Work out the finished part from the listing and answer in its coordinate system (mm). Coordinates: 2 decimals unless noted, no trailing zeros. Order: outer loops, then holes, each group sorted by start corner. A loop starts at its lowest first (then second) coordinate and runs counter-clockwise, first axis right, second up. Notation, with made-up numbers: (65.5, -9) -> (115.5, -9) arc R12 ccw to (115.5, -2) -> close; hole circle Ø11 at (64.25, 3.5). An arc over 180 degrees is marked (long way). Write item = value, one per line. Start each with the question number.
Q1. Flat-ended cylindrical pins translate along their axes: pin 1 (5 mm diameter, centred on y = 52, z = 9, fed in from +X); pin 2 (6 mm diameter, centred on x = 43.5, y = -23, fed in from -Z); pin 3 (3 mm diameter, centred on x = 52.5, z = 9.5, fed in from +Y); pin 4 (7.5 mm diameter, centred on y = 58.5, z = 7.5, fed in from +X). Find the tip coordinate at first contact, or state that the pin passes through.
Q2. Straight lines are drawn through the part: L1, parallel to X at y = -16, z = 5; L2, parallel to Y at x = 8, z = 11; L3, parallel to Y at x = 56, z = 4. For each, find the intervals that lie inside material, in ascending order. Write a range as from..to.
Q3. The part is cut by section A-A, the plane z = 2.75. Count the separate pieces of the cut face and the enclosed holes in it, plus the area to 3 significant figures.
Q4. For a pull along X with two mould halves and no side action, classify faces 1 (the flat face through (40.004, -48.798, 6.261)), 2 (the flat face through (16, 1, 12.7)), 3 (the flat face through (-12.11, -6.2, 6.26)) as +X half, -X half, draft (parallel to the pull), parting line (faces both ways), or undercut.
Q5. The part is cut by section C-C, the plane y = 33.5. Determine the outline of the cut face in (x, z).
Q6. The part is cut by section B-B, the plane x = -16.5. Determine the outline of the cut face in (y, z), plus the area to 3 significant figures.
```python
from build123d import *

# Parameters (mm, degrees)
F0_R     = 76.4587467439
F1_DEPTH = 12.7


with BuildPart() as f1:
    # F0 (on Top) → F1 (new body)
    with BuildSketch(Plane.XY):
        Circle(F0_R)
        with BuildLine():
            ThreePointArc((0, 67.8734653551), (47.9937876152, 47.9937876152), (67.8734653551, 0))
            ThreePointArc((67.8734653551, 0), (-31.0463451655, -60.3567042769), (-39.4713337388, 55.2161309057))
            Line((-39.4713337388, 55.2161309057), (-39.3394193415, 55.5124154929))
            Line((-39.3394193415, 55.5124154929), (-39.0032717993, 55.5477460232))
            ThreePointArc((-39.0032717993, 55.5477460232), (-20.4522527371, 64.7187195276), (0, 67.8734653551))
        make_face(mode=Mode.SUBTRACT)
        with BuildLine():
            ThreePointArc((-39.4713337388, 55.2161309057), (-31.0463451655, -60.3567042769), (67.8734653551, 0))
            ThreePointArc((67.8734653551, 0), (47.9937876152, 47.9937876152), (0, 67.8734653551))
            ThreePointArc((0, 67.8734653551), (-20.4522527371, 64.7187195276), (-39.0032717993, 55.5477460232))
            Line((-39.0032717993, 55.5477460232), (-29.885018528, 56.5061130603))
            Line((-29.885018528, 56.5061130603), (-24.2972507842, 48.8152105619))
            Line((-24.2972507842, 48.8152105619), (-28.1638838539, 40.1306104961))
            Line((-28.1638838539, 40.1306104961), (-37.6182846674, 39.1369129287))
            Line((-37.6182846674, 39.1369129287), (-43.2060524113, 46.8278154271))
            Line((-43.2060524113, 46.8278154271), (-39.4713337388, 55.2161309057))
        make_face()
        Polygon((-30.9335204728, -53.4327342282), (-40.3879212864, -52.4390366608), (-44.2545543561, -43.754436595), (-38.6667866123, -36.0635340966), (-29.2123857987, -37.057231664), (-25.345752729, -45.7418317298), align=None, mode=Mode.SUBTRACT)
        Polygon((6.9368320268, -60.8086286285), (-1.2960196783, -65.5618677767), (-9.5288713835, -60.8086286285), (-9.5288713835, -51.3021503321), (-1.2960196783, -46.548911184), (6.9368320268, -51.3021503321), align=None, mode=Mode.SUBTRACT)
        Polygon((-57.235837277, -25.2058756113), (-64.3005274315, -18.8448000245), (-62.3240194552, -9.5460610875), (-53.2828213244, -6.6083977373), (-46.21813117, -12.969473324), (-48.1946391463, -22.268212261), align=None, mode=Mode.SUBTRACT)
        Polygon((41.9100327329, -44.5162178486), (38.0433996632, -53.2008179144), (28.5889988496, -54.1945154818), (23.0012311058, -46.5036129834), (26.8678641755, -37.8190129176), (36.3222649891, -36.8253153502), align=None, mode=Mode.SUBTRACT)
        Polygon((60.6275076712, -10.7786490478), (62.6040156475, -20.0773879848), (55.539325493, -26.4384635716), (46.4981273623, -23.5008002214), (44.521619386, -14.2020612844), (51.5863095404, -7.8409856976), align=None, mode=Mode.SUBTRACT)
        Polygon((-61.9235273495, 13.0902466263), (-63.9000353258, 22.3889855633), (-56.8353451714, 28.7500611501), (-47.7941470406, 25.8123977998), (-45.8176390643, 16.5136588628), (-52.8823292188, 10.1525832761), align=None, mode=Mode.SUBTRACT)
        Polygon((4.2561218167, 13.0989960474), (8.0956247758, 11.1426715763), (11.1426715763, 8.0956247758), (13.0989960474, 4.2561218167), (13.7730995193, 0), (13.0989960474, -4.2561218167), (11.1426715763, -8.0956247758), (8.0956247758, -11.1426715763), (4.2561218167, -13.0989960474), (0, -13.7730995193), (-4.2561218167, -13.0989960474), (-8.0956247758, -11.1426715763), (-11.1426715763, -8.0956247758), (-13.0989960474, -4.2561218167), (-13.7730995193, 0), (-13.0989960474, 4.2561218167), (-11.1426715763, 8.0956247758), (-8.0956247758, 11.1426715763), (-4.2561218167, 13.0989960474), (0, 13.7730995193), align=None, mode=Mode.SUBTRACT)
        Polygon((55.9398175987, 27.5174731897), (63.0045077531, 21.156397603), (61.0279997768, 11.857658666), (51.9868016461, 8.9199953157), (44.9221114916, 15.2810709025), (46.8986194679, 24.5798098395), align=None, mode=Mode.SUBTRACT)
        Polygon((29.6375007945, 55.7443318067), (39.091901608, 54.7506342393), (42.9585346778, 46.0660341735), (37.3707669339, 38.3751316751), (27.9163661204, 39.3688292425), (24.0497330506, 48.0534293083), align=None, mode=Mode.SUBTRACT)
        Polygon((-8.2328517052, 63.1202262069), (0, 67.8734653551), (8.2328517052, 63.1202262069), (8.2328517052, 53.6137479106), (0, 48.8605087624), (-8.2328517052, 53.6137479106), align=None, mode=Mode.SUBTRACT)
    extrude(amount=F1_DEPTH)


solid = f1.part
```
Model answer:
q1.pin_1 = 58.27
q1.pin_2 = 0
q1.pin_3 = 56.96
q1.pin_4 = 53.37
q2.L1 = -74.77..-63.7, -46.86..44.9, 61.74..74.77
q2.L2 = -76.04..-11.19, 11.19..53.48, 63.25..76.04
q2.L3 = -52.06..-26.02, -9.28..10.22, 27.46..52.06
q3.separate_pieces = 1
q3.enclosed_holes = 11
q3.area = 15,400 mm2
q4.face_1 = undercut
q4.face_2 = draft
q4.face_3 = undercut
q5.outline = (-68.73, 0) -> (68.73, 0) -> (68.73, 12.7) -> (-68.73, 12.7) -> close
q6.outline = (-74.66, 0) -> (74.66, 0) -> (74.66, 12.7) -> (-74.66, 12.7) -> close
q6.area = 1,900 mm2
